Verification items for the finished model (mm, model axes). Face numbers are marked on the shaded views. A direction names the side the tool comes from. Coordinates: 2 decimals unless noted, no trailing zeros. Order: outer loops, then holes, each group sorted by start corner. A loop starts at its lowest first (then second) coordinate and runs counter-clockwise, first axis right, second up. Notation, with made-up numbers: M 51.5,50 L 107.5,50 A17 cw 107.5,62 Z; hole C 85,-34.5 d5. An arc over 180 degrees is marked long. Return JSON: item names as keys, results as strings.
```python
from build123d import *

# Parameters (mm, degrees)
BOSS_EXTRUDE1_DEPTH       = 7
HOLE3_START               = 3
HOLE3_OUTLINE_R           = 10.425
HOLE3_DEPTH               = 4
F_2_0MM_DOWEL_HOLE1_D     = 2
F_2_0MM_DOWEL_HOLE1_DEPTH = 7
F_2_0MM_DOWEL_HOLE1_TIP   = 0.600860619
F_1_5MM_DOWEL_HOLE1_D     = 1.5
F_1_5MM_DOWEL_HOLE1_DEPTH = 7
F_1_5MM_DOWEL_HOLE1_TIP   = 0.450645464


# Read off the part's stored shape, not the designer's step: Hole3
with BuildPart() as part:
    # Sketch1 → Boss-Extrude1 (new body)
    with BuildSketch(Plane(origin=(0, 0, 0), x_dir=(1, 0, 0), z_dir=(0, 1, 0))):
        with BuildLine():
            Line((0, 26), (0, 0))
            Line((0, 0), (35, 0))
            ThreePointArc((35, 0), (22, 13), (35, 26))
            Line((35, 26), (0, 26))
        make_face()
        with BuildLine():
            ThreePointArc((35, 26), (22, 13), (35, 0))
            Line((35, 0), (35, 26))
        make_face()
        with BuildLine():
            Line((35, 26), (35, 0))
            ThreePointArc((35, 0), (44.192388155, 3.807611845), (48, 13))
            ThreePointArc((48, 13), (44.192388155, 22.192388155), (35, 26))
        make_face()
    extrude(amount=BOSS_EXTRUDE1_DEPTH)

    # Hole3 outline → Hole3 (cut)
    with BuildSketch(Plane(origin=(0, 0, 0), x_dir=(1, 0, 0), z_dir=(0, 1, 0)).offset(HOLE3_START)):
        with Locations((35.011233351, 13.001482521)):
            Circle(HOLE3_OUTLINE_R)
    extrude(amount=HOLE3_DEPTH, mode=Mode.SUBTRACT)

    # Ø2.0mm Dowel Hole1
    with Locations(Plane(origin=(0, 0, 0), x_dir=(-1, 0, 0), z_dir=(0, -1, 0))):
        with Locations((-2.5, 6.5), (-2.5, 13), (-2.5, 19.5)):
            Hole(F_2_0MM_DOWEL_HOLE1_D / 2, depth=F_2_0MM_DOWEL_HOLE1_DEPTH)
            with Locations((0, 0, -(F_2_0MM_DOWEL_HOLE1_DEPTH + F_2_0MM_DOWEL_HOLE1_TIP / 2))):  # 118° drill point
                Cone(0, F_2_0MM_DOWEL_HOLE1_D / 2, F_2_0MM_DOWEL_HOLE1_TIP, mode=Mode.SUBTRACT)

    # Ø1.5mm Dowel Hole1
    with Locations(Plane(origin=(35, 0, -5.85), x_dir=(0, 0, -1), z_dir=(0, -1, 0))):
        with Locations((0, 0), (0, 3), (0, -3), (4.15, -7.15), (7.15, -7.15), (10.15, -7.15), (4.15, 7.15), (7.15, 7.15), (10.15, 7.15), (14.3, 0), (14.3, -3), (14.3, 3)):
            Hole(F_1_5MM_DOWEL_HOLE1_D / 2, depth=F_1_5MM_DOWEL_HOLE1_DEPTH)
            with Locations((0, 0, -(F_1_5MM_DOWEL_HOLE1_DEPTH + F_1_5MM_DOWEL_HOLE1_TIP / 2))):  # 118° drill point
                Cone(0, F_1_5MM_DOWEL_HOLE1_D / 2, F_1_5MM_DOWEL_HOLE1_TIP, mode=Mode.SUBTRACT)


solid = part.part
```
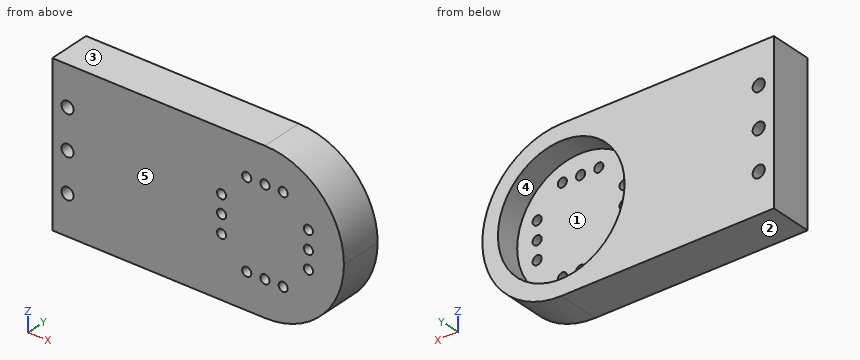
Q1. Cross-section at A-A, the plane x = 2.5. Record the boundary of the cut face in (y, z).
Values:
{"outline": "M 0,-26 L 7,-26 L 7,-20.5 L 0,-20.5 Z; M 0,-18.5 L 7,-18.5 L 7,-14 L 0,-14 Z; M 0,-12 L 7,-12 L 7,-7.5 L 0,-7.5 Z; M 0,-5.5 L 7,-5.5 L 7,0 L 0,0 Z"}
Q2. Cross-section at B-B, the plane y = 1.75. State how many separate pieces and enclosed holes the cut face has, and give its area (3 significant figures).
Values:
{"separate pieces": "1", "enclosed holes": "15", "area": "1,140 mm^2"}
Q3. Material ranges on line 1 along Z through (x, y) = (32, 1.65); line 2 along X through (y, z) = (1.1, -13); line 3 along Z through (x, y) = (2.5, 4.5), recorded low to high.
Values:
{"line 1": "-26 to -20.9, -19.4 to -6.6, -5.1 to 0", "line 2": "0 to 1.5, 3.5 to 27.1, 28.6 to 41.4, 42.9 to 48", "line 3": "-26 to -20.5, -18.5 to -14, -12 to -7.5, -5.5 to 0"}
Q4. Cross-section at D-D, the plane x = 38. Record the boundary of the cut face in (y, z), and give its area (3 significant figures).
Values:
{"outline": "M 0,-25.65 L 7,-25.65 L 7,-22.99 L 3,-22.99 L 3,-20.9 L 0,-20.9 Z; M 0,-19.4 L 3,-19.4 L 3,-6.6 L 0,-6.6 Z; M 0,-5.1 L 3,-5.1 L 3,-3.01 L 7,-3.01 L 7,-0.35 L 0,-0.35 Z", "area": "88.2 mm^2"}
Q5. Draft check along Z on the marked faces 1, 2 and 3. Enter one of: pulls with the +Z half, pulls with the -Z half, needs draft (parallel to the pull), parting line crosses it, or undercut.
Values:
{"face 1": "undercut", "face 2": "pulls with the -Z half", "face 3": "pulls with the +Z half"}
Q6. Go/stop test with flat-tipped pins: pin 1 (2 mm diameter, centred on x = 38, z = -20.15, fed in from -Y); pin 2 (2.5 mm diameter, centred on x = 27.85, z = -10, fed in from +Y). Record where each tip stops, or that it passes through.
Values:
{"pin 1": "y = 0", "pin 2": "y = 3"}
Q7. Tool access check on the marked faces 4 and 5. Record the directions out of +Z, -Z, +X, -X, +Y, -Y that give a thin tool (end or side, any length) a straight path to the whole face; none if there is none.
Values:
{"face 4": "+Y", "face 5": "+Z, -Z, +X, -X, -Y"}
Q8. Cross-section at C-C, the plane z = -10. Record the boundary of the cut face in (x, y), and give its area (3 significant figures).
Values:
{"outline": "M 0,0 L 27.1,0 L 27.1,3 L 25.03,3 L 25.03,7 L 0,7 Z; M 28.6,0 L 41.4,0 L 41.4,3 L 28.6,3 Z; M 42.9,0 L 47.65,0 L 47.65,7 L 44.99,7 L 44.99,3 L 42.9,3 Z", "area": "245 mm^2"}
